CAD build for the part. Positions are in the model's coordinates, mm. Face numbers are marked on the shaded views. Give positions to 0.01 mm unless a question says otherwise; leave off trailing zeros. Loops run counter-clockwise (first coordinate to the right, second up) from the corner with the lowest first, then second, coordinate; pieces in that order, holes last.
Item 1: Mould opens along Y. For the marked faces 1 and 2 say: released by +Y, released by -Y, zero draft, split by the parting line, or undercut.
Item 2: Probe probe 1 along X at (y, z) = (-6.25, 0.3); probe 2 along X at (y, z) = (-7.25, 0.3); probe 3 along Z at (x, y) = (-13, -4). List the from-to ranges inside material, lowest first.
Item 3: Saw through at C-C on x = -4.75. Give the cut face in (y, z).
Item 4: Saw through at B-B on x = -8. Give the cut face in (y, z).
Item 5: Saw through at A-A on z = 0.1. Give the cut face in (x, y), plus the area to 3 significant figures.
Item 6: Saw through at D-D on x = -11. Give the cut face in (y, z).
from build123d import *

# Parameters (mm, degrees)
EXTRUSION1_DEPTH = 0.2
ESQUISSE2_W      = 1.59785128
ESQUISSE2_H      = 1.03077013
ESQUISSE2_W_2    = 10.83121002
ESQUISSE2_H_2    = 0.3
EXTRUSION2_DEPTH = 0.2


with BuildPart() as part:
    # Esquisse1 → Extrusion1 (new body)
    with BuildSketch(Plane.XY):
        with BuildLine():
            Line((-27.5, -6.00142003), (-27.5, -8.00142003))
            ThreePointArc((-27.5, -8.00142003), (-26.914213562, -9.415633592), (-25.5, -10.00142003))
            Line((-25.5, -10.00142003), (-23.865139014, -10.00142003))
            ThreePointArc((-23.865139014, -10.00142003), (-23.210588236, -9.891278035), (-22.628130987, -9.572983309))
            ThreePointArc((-22.628130987, -9.572983309), (-14, -6.584637184), (-5.371869013, -9.572983309))
            ThreePointArc((-5.371869013, -9.572983309), (-4.789411764, -9.891278035), (-4.134860986, -10.00142003))
            Line((-4.134860986, -10.00142003), (-2.5, -10.00142003))
            ThreePointArc((-2.5, -10.00142003), (-1.085786438, -9.415633592), (-0.5, -8.00142003))
            Line((-0.5, -8.00142003), (-0.5, -6.00142003))
            ThreePointArc((-0.5, -6.00142003), (-1.964466094, -2.465886124), (-5.5, -1.00142003))
            Line((-5.5, -1.00142003), (-22.5, -1.00142003))
            ThreePointArc((-22.5, -1.00142003), (-26.035533906, -2.465886124), (-27.5, -6.00142003))
        make_face()
    extrude(amount=EXTRUSION1_DEPTH)

    # Esquisse2 → Extrusion2 (add)
    # profile 1 of 4: a face of its own
    with BuildSketch(Plane.XY.offset(0.2)):
        with BuildLine():
            Line((-14.730316635, -2.510657311), (-14.006042275, -2.510657311))
            Line((-14.006042275, -2.510657311), (-14.006042275, -2.111468697))
            ThreePointArc((-14.006042275, -2.111468697), (-14.066642884, -1.886467114), (-14.232049919, -1.722337108))
            ThreePointArc((-14.232049919, -1.722337108), (-15.798042275, -1.307063885), (-17.364034631, -1.722337108))
            ThreePointArc((-17.364034631, -1.722337108), (-17.529441665, -1.886467114), (-17.590042275, -2.111468697))
            Line((-17.590042275, -2.111468697), (-17.590042275, -2.510657311))
            Line((-17.590042275, -2.510657311), (-16.965767915, -2.510657311))
            Line((-16.965767915, -2.510657311), (-16.965767915, -3.541427441))
            Line((-16.965767915, -3.541427441), (-21.408442275, -3.541427441))
            Line((-21.408442275, -3.541427441), (-21.408442275, -3.841427441))
            Line((-21.408442275, -3.841427441), (-10.477242275, -3.859176516))
            Line((-10.477242275, -3.859176516), (-10.477242275, -3.541427441))
            Line((-10.477242275, -3.541427441), (-14.730316635, -3.541427441))
            Line((-14.730316635, -3.541427441), (-14.730316635, -2.510657311))
        make_face()
        with Locations((-15.798042275, -3.026042376)):
            Rectangle(ESQUISSE2_W, ESQUISSE2_H, mode=Mode.SUBTRACT)
        with BuildLine():
            Line((-17.321242275, -2.241857311), (-14.274842275, -2.241857311))
            Line((-14.274842275, -2.241857311), (-14.274842275, -2.111468697))
            ThreePointArc((-14.274842275, -2.111468697), (-14.299082519, -2.021468064), (-14.365245332, -1.955816061))
            ThreePointArc((-14.365245332, -1.955816061), (-15.798042275, -1.575863885), (-17.230839217, -1.955816061))
            ThreePointArc((-17.230839217, -1.955816061), (-17.297002031, -2.021468064), (-17.321242275, -2.111468697))
            Line((-17.321242275, -2.111468697), (-17.321242275, -2.241857311))
        make_face(mode=Mode.SUBTRACT)
    # profile 2 of 4: a face of its own
    with BuildSketch(Plane.XY.offset(0.2)):
        with Locations((-15.892837265, -5.434307441)):
            Rectangle(ESQUISSE2_W_2, ESQUISSE2_H_2)
    # profile 3 of 4: a face of its own
    with BuildSketch(Plane.XY.offset(0.2)):
        with BuildLine():
            Line((-11.983013473, -2.941427441), (-11.983013473, -2.637464752))
            Line((-11.983013473, -2.637464752), (-9.677242275, -2.637464752))
            Line((-9.677242275, -2.637464752), (-9.677242275, -3.559176516))
            Line((-9.677242275, -3.559176516), (-6.924787178, -3.559176516))
            ThreePointArc((-6.924787178, -3.559176516), (-4.435771308, -4.590160647), (-3.404787178, -7.079176516))
            Line((-3.404787178, -7.079176516), (-3.404787178, -8.399718672))
            Line((-3.404787178, -8.399718672), (-3.704787178, -8.399718672))
            Line((-3.704787178, -8.399718672), (-3.704787178, -7.079176516))
            ThreePointArc((-3.704787178, -7.079176516), (-4.647903343, -4.802292681), (-6.924787178, -3.859176516))
            Line((-6.924787178, -3.859176516), (-9.977242275, -3.859176516))
            Line((-9.977242275, -3.859176516), (-9.977242275, -2.941427441))
            Line((-9.977242275, -2.941427441), (-11.983013473, -2.941427441))
        make_face()
    # profile 4 of 4: a face of its own
    with BuildSketch(Plane.XY.offset(0.2)):
        with BuildLine():
            Line((-5.444787178, -7.079176516), (-5.444787178, -8.399718672))
            Line((-5.444787178, -8.399718672), (-5.144787178, -8.399718672))
            Line((-5.144787178, -8.399718672), (-5.144787178, -7.079176516))
            ThreePointArc((-5.144787178, -7.079176516), (-5.666137108, -5.820526446), (-6.924787178, -5.299176516))
            Line((-6.924787178, -5.299176516), (-9.977242275, -5.299176516))
            Line((-9.977242275, -5.299176516), (-9.977242275, -6.184307441))
            Line((-9.977242275, -6.184307441), (-11.983013473, -6.184307441))
            Line((-11.983013473, -6.184307441), (-11.983013473, -6.488270129))
            Line((-11.983013473, -6.488270129), (-9.677242275, -6.488270129))
            Line((-9.677242275, -6.488270129), (-9.677242275, -5.599176516))
            Line((-9.677242275, -5.599176516), (-6.924787178, -5.599176516))
            ThreePointArc((-6.924787178, -5.599176516), (-5.878269142, -6.03265848), (-5.444787178, -7.079176516))
        make_face()
    extrude(amount=EXTRUSION2_DEPTH)


solid = part.part
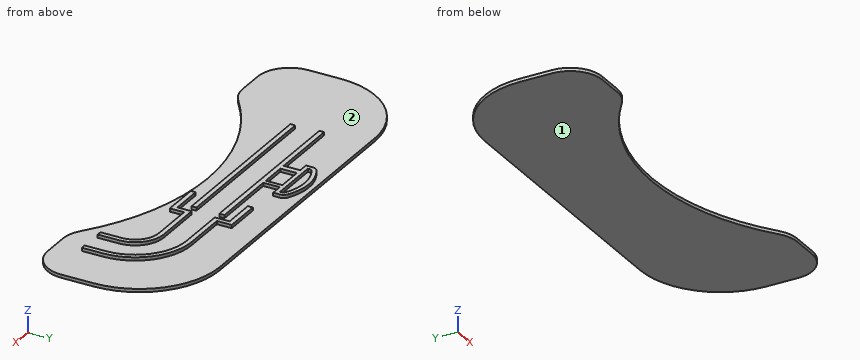
Results below:
1. face 1: zero draft
1. face 2: undercut
2. probe 1: x = -11.98 to -9.68, -5.7 to -5.35, -3.81 to -3.5
2. probe 2: x = -5.44 to -5.14, -3.7 to -3.4
2. probe 3: z = 0 to 0.2
3. outline: (-9.9, 0) - (-1.06, 0) - (-1.06, 0.2) - (-4.31, 0.2) - (-4.31, 0.4) - (-4.7, 0.4) - (-4.7, 0.2) - (-9.9, 0.2) - close
4. outline: (-7.94, 0) - (-1, 0) - (-1, 0.2) - (-3.56, 0.2) - (-3.56, 0.4) - (-3.86, 0.4) - (-3.86, 0.2) - (-5.3, 0.2) - (-5.3, 0.4) - (-5.6, 0.4) - (-5.6, 0.2) - (-7.94, 0.2) - close
5. outline: (-27.5, -8) arc R2 ccw to (-25.5, -10) - (-23.87, -10) arc R2 ccw to (-22.63, -9.57) arc R13.95 cw to (-5.37, -9.57) arc R2 ccw to (-4.13, -10) - (-2.5, -10) arc R2 ccw to (-0.5, -8) - (-0.5, -6) arc R5 ccw to (-5.5, -1) - (-22.5, -1) arc R5 ccw to (-27.5, -6) - close
5. area: 188 mm2
6. outline: (-6.91, 0) - (-1, 0) - (-1, 0.2) - (-2.64, 0.2) - (-2.64, 0.4) - (-2.94, 0.4) - (-2.94, 0.2) - (-3.54, 0.2) - (-3.54, 0.4) - (-3.86, 0.4) - (-3.86, 0.2) - (-5.28, 0.2) - (-5.28, 0.4) - (-5.58, 0.4) - (-5.58, 0.2) - (-6.18, 0.2) - (-6.18, 0.4) - (-6.49, 0.4) - (-6.49, 0.2) - (-6.91, 0.2) - close
